Geometry check sheet. Reference: the model listing, model coordinates, mm. A direction names the side the tool comes from. Coordinates: 2 decimals unless noted, no trailing zeros. Loops run counter-clockwise (first coordinate to the right, second up) from the corner with the lowest first, then second, coordinate; pieces in that order, holes last.
from build123d import *

# Parameters (mm, degrees)
SKETCH1_R           = 7.95
BOSS_EXTRUDE1_DEPTH = 48
SKETCH3_R           = 3.85
BOSS_EXTRUDE2_DEPTH = 15.9
BOSS_EXTRUDE3_START = 20
SKETCH8_R           = 3.85
BOSS_EXTRUDE3_DEPTH = 20
CUT_EXTRUDE2_DEPTH  = 15.1
SKETCH4_W           = 1
SKETCH4_H           = 91
CUT_EXTRUDE1_DEPTH  = 10


with BuildPart() as part:
    # Sketch1 → Boss-Extrude1 (new, symmetric)
    with BuildSketch(Plane.XY):
        Circle(SKETCH1_R)
    extrude(amount=BOSS_EXTRUDE1_DEPTH, both=True)

    # Sketch3 → Boss-Extrude2 (add)
    with BuildSketch(Plane.XY.offset(48)):
        Circle(SKETCH3_R)
    extrude(amount=BOSS_EXTRUDE2_DEPTH)

    # Sketch8 → Boss-Extrude3 (add)
    with BuildSketch(Plane(origin=(0, 0, -48), x_dir=(-1, 0, 0), z_dir=(0, 0, -1)).offset(BOSS_EXTRUDE3_START)):
        with Locations(Location((0, 0, 0), (0, 0, 180))):
            Circle(SKETCH8_R)
    extrude(amount=-BOSS_EXTRUDE3_DEPTH)

    # Sketch6 → Cut-Extrude2 (cut)
    with BuildSketch(Plane.XY.offset(63.9)):
        Polygon((-1.1, 2.6), (1.1, 2.6), (1.1, 1.1), (2.6, 1.1), (2.6, -1.1), (1.1, -1.1), (1.1, -2.6), (-1.1, -2.6), (-1.1, -1.1), (-2.6, -1.1), (-2.6, 1.1), (-1.1, 1.1), align=None)
    extrude(amount=-CUT_EXTRUDE2_DEPTH, mode=Mode.SUBTRACT)

    # Sketch4 → Cut-Extrude1 (cut)
    with BuildSketch(Plane(origin=(0, 7.95, 0), x_dir=(1, 0, 0), z_dir=(0, 1, 0))):
        Rectangle(SKETCH4_W, SKETCH4_H)
    extrude(amount=-CUT_EXTRUDE1_DEPTH, mode=Mode.SUBTRACT)


solid = part.part
1) Section check B-B on x = -6.75. Record the cut outline in (y, z).
Data:
outline: (-4.2, -48) - (4.2, -48) - (4.2, 48) - (-4.2, 48) - close
2) Section check D-D on y = 6. Record the cut outline in (x, z), and give its area (3 significant figures).
Data:
outline: (-5.22, -48) - (5.22, -48) - (5.22, 48) - (-5.22, 48) - close; hole (-0.5, -45.5) - (0.5, -45.5) - (0.5, 45.5) - (-0.5, 45.5) - close
area: 910 mm2
3) Depth check by flat-ended pin: pin 1 (6 mm diameter, centred on x = -4, y = -2.5, fed in from -Z); pin 2 (0.8 mm diameter, centred on y = 2, z = 57, fed in from +X); pin 3 (1.2 mm diameter, centred on x = 2, z = 53, fed in from +Y); pin 4 (3 mm diameter, centred on x = -3, z = 46.5, fed in from -Y). Enter the tip coordinate at first touch or a pass-through.
Data:
pin 1: stops at z = -68
pin 2: stops at x = 3.5
pin 3: stops at y = 3.59
pin 4: stops at y = -7.81
4) Section check A-A on y = 0. Record the cut outline in (x, z), and give its area (3 significant figures).
Data:
outline: (-7.95, -48) - (-3.85, -48) - (-3.85, -68) - (3.85, -68) - (3.85, -48) - (7.95, -48) - (7.95, 48) - (3.85, 48) - (3.85, 63.9) - (2.6, 63.9) - (2.6, 48.8) - (-2.6, 48.8) - (-2.6, 63.9) - (-3.85, 63.9) - (-3.85, 48) - (-7.95, 48) - close; hole (-0.5, -45.5) - (0.5, -45.5) - (0.5, 45.5) - (-0.5, 45.5) - close
area: 1,630 mm2
5) Material ranges on probe 1 along X at (y, z) = (-0.5, 30.5); probe 2 along Z at (x, y) = (0, 4.25); probe 3 along Z at (x, y) = (-1, 6.5), recorded low to high.
Data:
probe 1: x = -7.93 to -0.5, 0.5 to 7.93
probe 2: z = -48 to -45.5, 45.5 to 48
probe 3: z = -48 to 48
6) Mould release check, pull along Z, two halves, no side actions. Record for faces 1 (the flat face through (0, -2.6, 56)), 2 (the flat face through (-4, -2, -48)), 3 (the flat face through (-2, 2, 63.9)), 4 (the flat face through (-0.5, 3, 1)): +Z half, -Z half, draft (parallel to the pull), parting line (faces both ways), or undercut.
Data:
face 1: draft
face 2: -Z half
face 3: +Z half
face 4: undercut
7) Access from +Z, -Z, +X, -X, +Y, -Y to the whole of each face (thin tool, end or side, straight path). Record for faces 5 (the flat face through (0, 2.6, 56)), 6 (the flat face through (0.5, 3, 1)), 7 (the cylindrical face through (-0.83, 3.76, -58.14)), 8 (the flat face through (0, 0, -68)).
Data:
face 5: +Z
face 6: +Y
face 7: -Z
face 8: -Z, +X, -X, +Y, -Y
8) Section check C-C on z = 17. Record the cut outline in (x, y).
Data:
outline: (-0.5, -2.05) - (-0.5, 7.93) arc R7.95 ccw (long way) to (0.5, 7.93) - (0.5, -2.05) - close
